from build123d import *

# Parameters (mm, degrees)
MAIN_BODY_SKETCH_R     = 117.99951
MAIN_BODY_DEPTH        = 3.175
TABS_SKETCH_W          = 6.35
TABS_SKETCH_H          = 152.4
TABS_SKETCH_W_2        = 152.4
TABS_SKETCH_H_2        = 6.35
OUTSIDE_TABS_DEPTH     = 6.35
F_6_0_204_TUBE_MOUNT_D = 5.1816
SKETCH12_W             = 165.1
SKETCH12_H             = 50.8
BOSS_EXTRUDE1_DEPTH    = 6.35
SKETCH13_R             = 1.5
CUT_EXTRUDE1_DEPTH     = 489.042014073
SKETCH14_W             = 6.35
SKETCH14_H             = 12.7
CUT_EXTRUDE2_DEPTH     = 489.042014073
SKETCH15_W             = 87.70313901
SKETCH15_H             = 6.35
CUT_EXTRUDE3_DEPTH     = 489.042014073
SKETCH16_W             = 34.925
SKETCH16_H             = 34.925
CUT_EXTRUDE4_DEPTH     = 489.042014073
SKETCH17_W             = 158.75
SKETCH17_H             = 10.820932089
CUT_EXTRUDE5_DEPTH     = 489.042014073
FILLET1_R              = 25.4


with BuildPart() as part:
    # Main Body Sketch → Main Body (new, symmetric)
    with BuildSketch(Plane.XY):
        with BuildLine():
            Line((-96.545932089, -95.25), (-254, -95.25))
            Line((-254, -95.25), (-254, 95.25))
            Line((-254, 95.25), (-96.545932089, 95.25))
            ThreePointArc((-96.545932089, 95.25), (0, 135.6233), (96.545932089, 95.25))
            Line((96.545932089, 95.25), (254, 95.25))
            Line((254, 95.25), (254, -95.25))
            Line((254, -95.25), (96.545932089, -95.25))
            ThreePointArc((96.545932089, -95.25), (95.900155117, -95.900155117), (95.25, -96.545932089))
            Line((95.25, -96.545932089), (95.25, -406.4))
            Line((95.25, -406.4), (-95.25, -406.4))
            Line((-95.25, -406.4), (-95.25, -96.545932089))
            ThreePointArc((-95.25, -96.545932089), (-95.900155117, -95.900155117), (-96.545932089, -95.25))
        make_face()
        Circle(MAIN_BODY_SKETCH_R, mode=Mode.SUBTRACT)
    extrude(amount=MAIN_BODY_DEPTH, both=True)

    # Tabs Sketch → Outside Tabs (add)
    with BuildSketch(Plane.XY.offset(3.175)):
        with Locations((-257.175, 0)):
            Rectangle(TABS_SKETCH_W, TABS_SKETCH_H)
        with Locations((0, -409.575)):
            Rectangle(TABS_SKETCH_W_2, TABS_SKETCH_H_2)
    outside_tabs = extrude(amount=-OUTSIDE_TABS_DEPTH)

    # Outside Tabs Mirror: Outside Tabs across plane
    add(outside_tabs.mirror(Plane(origin=(0, 0, 0), x_dir=(0, 0, 1), z_dir=(1, 0, 0))))

    # #6 (0.204) Tube Mount (through all)
    with Locations(Plane.XY.offset(3.175)):
        with Locations((0, -123.19), (123.19, 0), (0, 123.19), (-123.19, 0)):
            Hole(F_6_0_204_TUBE_MOUNT_D / 2)

    # Sketch12 → Boss-Extrude1 (add)
    with BuildSketch(Plane.XY.offset(3.175)):
        with Locations((-177.8, -342.9)):
            Rectangle(SKETCH12_W, SKETCH12_H)
        with Locations((177.8, -342.9)):
            Rectangle(SKETCH12_W, SKETCH12_H)
    extrude(amount=-BOSS_EXTRUDE1_DEPTH)

    # Sketch13 → Cut-Extrude1 (cut, through all)
    with BuildSketch(Plane.XY.offset(3.175)):
        with Locations((-196.85, -333.4)):
            Circle(SKETCH13_R)
        with Locations((-187.35, -342.9)):
            Circle(SKETCH13_R)
        with Locations((-196.85, -352.4)):
            Circle(SKETCH13_R)
        with Locations((-206.35, -342.9)):
            Circle(SKETCH13_R)
    cut_extrude1 = extrude(amount=-CUT_EXTRUDE1_DEPTH, mode=Mode.SUBTRACT)

    # Mirror2: Cut-Extrude1 across plane
    add(cut_extrude1.mirror(Plane(origin=(0, 0, 0), x_dir=(0, 0, 1), z_dir=(1, 0, 0))), mode=Mode.SUBTRACT)

    # Sketch14 → Cut-Extrude2 (cut, through all)
    with BuildSketch(Plane.XY.offset(3.175)):
        with Locations((-257.175, -323.85)):
            Rectangle(SKETCH14_W, SKETCH14_H)
        with Locations((-257.175, -361.95)):
            Rectangle(SKETCH14_W, SKETCH14_H)
    cut_extrude2 = extrude(amount=-CUT_EXTRUDE2_DEPTH, mode=Mode.SUBTRACT)

    # Mirror3: Cut-Extrude2 across plane
    add(cut_extrude2.mirror(Plane(origin=(0, 0, 0), x_dir=(0, 0, 1), z_dir=(1, 0, 0))), mode=Mode.SUBTRACT)

    # Sketch15 → Cut-Extrude3 (cut, through all)
    with BuildSketch(Plane.XY.offset(3.175)):
        with Locations((-133.948430495, -73.025)):
            Rectangle(SKETCH15_W, SKETCH15_H)
        with Locations((133.948430495, -73.025)):
            Rectangle(SKETCH15_W, SKETCH15_H)
    extrude(amount=-CUT_EXTRUDE3_DEPTH, mode=Mode.SUBTRACT)

    # Sketch16 → Cut-Extrude4 (cut, through all)
    with BuildSketch(Plane.XY.offset(3.175)):
        with Locations((134.162737592, 0)):
            Rectangle(SKETCH16_W, SKETCH16_H)
    cut_extrude4 = extrude(amount=-CUT_EXTRUDE4_DEPTH, mode=Mode.SUBTRACT)

    # Mirror4: Cut-Extrude4 across plane
    add(cut_extrude4.mirror(Plane(origin=(0, 0, 0), x_dir=(0, 0, 1), z_dir=(1, 0, 0))), mode=Mode.SUBTRACT)

    # Sketch17 → Cut-Extrude5 (cut, through all)
    with BuildSketch(Plane.XY.offset(3.175)):
        with Locations((-174.625, -91.135466045)):
            Rectangle(SKETCH17_W, SKETCH17_H)
    cut_extrude5 = extrude(amount=-CUT_EXTRUDE5_DEPTH, mode=Mode.SUBTRACT)

    # Mirror5: Cut-Extrude5 across plane
    add(cut_extrude5.mirror(Plane(origin=(0, 0, 0), x_dir=(0, 0, 1), z_dir=(1, 0, 0))), mode=Mode.SUBTRACT)

    # Fillet1
    fillet1_edges = [part.edges().sort_by_distance(p)[0] for p in [
        (-95.25, -317.5, 0),
        (-95.25, -368.3, 0),
        (95.25, -317.5, 0),
        (95.25, -368.3, 0),
        (-96.545932089, 95.25, 0),
        (96.545932089, 95.25, 0),
        (-95.25, -85.725, 0),
        (95.25, -85.725, 0),
    ]]
    fillet(fillet1_edges, radius=FILLET1_R)


solid = part.part
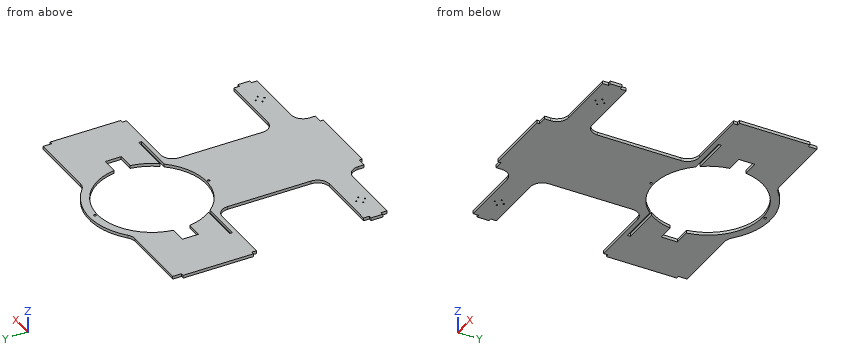
Work out the finished part from the listing and answer in its coordinate system (mm). Give positions to 0.01 mm unless a question says otherwise; leave off trailing zeros. Order: outer loops, then holes, each group sorted by start corner. A loop starts at its lowest first (then second) coordinate and runs counter-clockwise, first axis right, second up. Notation, with made-up numbers: (-32, -17.5) - (-14, -17.5) arc R12 ccw to (-14, -10.5) - close; hole circle Ø1 at (58.5, -11). An arc over 180 degrees is marked (long way). Answer as CSV lines item,"result". Start each with the question number.
Q1. The part is cut by section C-C (y = -278). Write down the section's boundary in (x, z) (3 decimals).
Q2. The part is cut by section D-D (x = -40). Write down the section's boundary in (y, z) (3 decimals), then the cut area to 3 significant figures.
Q3. Given pin 1 Ø1.8 at (x, y) = (-196.85, -352.4) entering from +Z; pin 2 Ø1.9 at (x, z) = (-258, 1.5) entering from +Y; pin 3 Ø1.9 at (y, z) = (87.5, 1) entering from -X; pin 4 Ø1.9 at (y, z) = (85, 0) entering from +X, each flat-ended and moving along its own axis, determine where each tip first touches the part or whether it passes through.
Q4. Find the intervals of material crossed by L1, parallel to X at y = -333.4, z = -1.5; L2, parallel to X at y = -342.9, z = -1.5; L3, parallel to Y at x = -196.85, z = -0.25 (3 decimals), in increasing order. Write a range as [from, to].
Q5. The part is cut by section B-B (z = -0.25). Give the number of separate pieces and of enclosed holes in the cut face, then the cut area to 3 significant figures.
Q6. The part is cut by section A-A (x = -218.5). Write down the section's boundary in (y, z) (3 decimals), then the cut area to 3 significant figures.
Check result:
1,outline,"(-95.25, -3.175) - (95.25, -3.175) - (95.25, 3.175) - (-95.25, 3.175) - close"
2,outline,"(-412.75, -3.175) - (-111.013, -3.175) - (-111.013, 3.175) - (-412.75, 3.175) - close; (111.013, -3.175) - (129.59, -3.175) - (129.59, 3.175) - (111.013, 3.175) - close"
2,area,"2,030 mm²"
3,pin 1,"passes through"
3,pin 2,"stops at y = 76.2"
3,pin 3,"stops at x = -254"
3,pin 4,"stops at x = 254"
4,L1,"x = [-260.35, -198.35], [-195.35, 195.35], [198.35, 260.35]"
4,L2,"x = [-260.35, -207.85], [-204.85, -188.85], [-185.85, 185.85], [188.85, 204.85], [207.85, 260.35]"
4,L3,"y = [-368.3, -353.9], [-350.9, -334.9], [-331.9, -317.5], [-85.725, 95.25]"
5,separate pieces,"1"
5,enclosed holes,"11"
5,area,"131,000 mm²"
6,outline,"(-368.3, -3.175) - (-317.5, -3.175) - (-317.5, 3.175) - (-368.3, 3.175) - close; (-85.725, -3.175) - (95.25, -3.175) - (95.25, 3.175) - (-85.725, 3.175) - close"
6,area,"1,470 mm²"
